Verification items for the finished model (mm, model axes). A direction names the side the tool comes from. Round coordinates to 2 decimals unless told otherwise and drop trailing zeros. Order: outer loops, then holes, each group sorted by start corner. A loop starts at its lowest first (then second) coordinate and runs counter-clockwise, first axis right, second up. Notation, with made-up numbers: (46.25, -11.5) -> (63.25, -11.5) arc R9 ccw to (63.25, 1.5) -> close; hole circle Ø3 at (20, 28). An arc over 180 degrees is marked (long way). Return JSON: item names as keys, results as strings. Group by question number.
Item 1: Access from +Z, -Z, +X, -X, +Y, -Y to the whole of each face (thin tool, end or side, straight path). Record for faces 1 (the cylindrical face through (-48, 18, 0)), 2 (the flat face through (20, 0, 0)), 3 (the flat face through (38, 13, 0)), 4 (the flat face through (-35.2, 13, 0.3)), 5 (the cylindrical face through (-22.5, 23, 0.1)).
Item 2: Sectioned sample at B-B on y = 21. Record the cut outline in (x, z), plus the area to 3 significant figures.
Item 3: Depth check by flat-ended pin: pin 1 Ø6.5 at (x, z) = (-31, 0) entering from -Y; pin 2 Ø4 at (y, z) = (6.5, 5.5) entering from -X; pin 3 Ø6.5 at (y, z) = (6, -3.5) entering from +X; pin 4 Ø5.5 at (x, z) = (0, 0) entering from +Y (3 decimals). Enter the tip coordinate at first touch or a pass-through.
Item 4: Sectioned sample at A-A on x = 31. Record the cut outline in (y, z), plus the area to 3 significant figures.
Item 5: Sectioned sample at C-C on y = 7.5. Record the cut outline in (x, z), plus the area to 3 significant figures.
Item 6: Draft check along X on faces 6 (the cylindrical face through (2.93, 25.59, -0.65)), 7 (the cylindrical face through (22.5, 23, 0.1)), 8 (the flat face through (-38, 22, 0)). Enter one of: pulls with the +X half, pulls with the -X half, needs draft (parallel to the pull), parting line crosses it, or undercut.
Item 7: Sectioned sample at D-D on z = 0. Give the number of separate pieces and of enclosed holes in the cut face, plus the area to 3 significant figures.
Item 8: Scan lines: probe 1 along Z at (x, y) = (-31, 16); probe 2 along X at (y, z) = (24.25, 0); probe 3 along Y at (x, z) = (40.5, 1). Record each from-to range of solid material in increasing order. Write a range as from..to.
```python
from build123d import *

# Parameters (mm, degrees)
BOSS_EXTRUDE1_DEPTH   = 18
F_8_0MM_DOWEL_HOLE1_D = 8
CUT_EXTRUDE1_DEPTH    = 36
CUT_EXTRUDE4_DEPTH    = 36


with BuildPart() as part:
    # Sketch2 → Boss-Extrude1 (new body, symmetric)
    with BuildSketch(Plane.XY):
        with BuildLine():
            Line((18.027756377, 0), (22, 0))
            Line((22, 0), (22, 13))
            Line((22, 13), (50, 13))
            Line((50, 13), (50, 22))
            Line((50, 22), (25.690465157, 22))
            ThreePointArc((25.690465157, 22), (0, 32), (-25.690465157, 22))
            Line((-25.690465157, 22), (-50, 22))
            Line((-50, 22), (-50, 13))
            Line((-50, 13), (-22, 13))
            Line((-22, 13), (-22, 0))
            Line((-22, 0), (-18.027756377, 0))
            ThreePointArc((-18.027756377, 0), (0, 13), (18.027756377, 0))
        make_face()
    extrude(amount=BOSS_EXTRUDE1_DEPTH, both=True)

    # Ø8.0mm Dowel Hole1 (through all)
    with Locations(Plane(origin=(0, 22, 0), x_dir=(1, 0, 0), z_dir=(0, 1, 0))):
        with Locations((-31, 0)):
            f_8_0mm_dowel_hole1 = Hole(F_8_0MM_DOWEL_HOLE1_D / 2)

    # Sketch9 → Cut-Extrude1 (cut)
    with BuildSketch(Plane(origin=(0, 22, 0), x_dir=(1, 0, 0), z_dir=(0, 1, 0))):
        with BuildLine():
            ThreePointArc((-44.497190923, -18), (-48, 0), (-44.497190923, 18))
            Line((-44.497190923, 18), (-50, 18))
            Line((-50, 18), (-50, -18))
            Line((-50, -18), (-44.497190923, -18))
        make_face()
    cut_extrude1 = extrude(amount=-CUT_EXTRUDE1_DEPTH, mode=Mode.SUBTRACT)

    # Mirror1: Ø8.0mm Dowel Hole1, Cut-Extrude1 across plane
    add(f_8_0mm_dowel_hole1.mirror(Plane(origin=(0, 0, 0), x_dir=(0, 0, 1), z_dir=(1, 0, 0))), mode=Mode.SUBTRACT)
    add(cut_extrude1.mirror(Plane(origin=(0, 0, 0), x_dir=(0, 0, 1), z_dir=(1, 0, 0))), mode=Mode.SUBTRACT)

    # Sketch10 → CBORE for M5 Hex Head Bolt1 (revolve, cut)
    with BuildSketch(Plane(origin=(0, 32, 0), x_dir=(0, 0, 1), z_dir=(1, 0, 0))):
        Polygon((0, 0), (0, 32), (2.5, 32), (2.5, 13.495), (2.995, 13), (3, 13), (3, 0), align=None)
    revolve(axis=Axis((0, 38.35, 0), (0, -1, 0)), mode=Mode.SUBTRACT)

    # Sketch12 → Cut-Extrude4 (cut)
    with BuildSketch(Plane(origin=(0, 22, 0), x_dir=(1, 0, 0), z_dir=(0, 1, 0))):
        with BuildLine():
            Line((-25.690465157, 6.637683312), (-25.690465157, -6.637683312))
            ThreePointArc((-25.690465157, -6.637683312), (-22.5, 0), (-25.690465157, 6.637683312))
        make_face()
    cut_extrude4 = extrude(amount=CUT_EXTRUDE4_DEPTH, mode=Mode.SUBTRACT)

    # Mirror2: Cut-Extrude4 across plane
    add(cut_extrude4.mirror(Plane(origin=(0, 0, 0), x_dir=(0, 0, 1), z_dir=(1, 0, 0))), mode=Mode.SUBTRACT)


solid = part.part
```
Recorded:
{
 "1": {"face 1": "-X, +Y, -Y", "face 2": "+Z, -Z, +X, -X, -Y", "face 3": "+Z, -Z, +X, -Y", "face 4": "+Z, -Z, -X, -Y", "face 5": "-X, +Y"},
 "2": {"outline": "(-44.5, -18) -> (44.5, -18) arc R48 ccw to (44.5, 18) -> (-44.5, 18) arc R48 ccw to start; hole circle Ø8 at (-31, 0); hole circle Ø6 at (0, 0); hole circle Ø8 at (31, 0)", "area": "3,240 mm²"},
 "3": {"pin 1": "through", "pin 2": "x = -22", "pin 3": "x = 22", "pin 4": "y = 18.755"},
 "4": {"outline": "(13, -18) -> (22, -18) -> (22, -4) -> (13, -4) -> close; (13, 4) -> (22, 4) -> (22, 18) -> (13, 18) -> close", "area": "252 mm²"},
 "5": {"outline": "(-22, -18) -> (-13.37, -18) -> (-13.37, 18) -> (-22, 18) -> close; (13.37, -18) -> (22, -18) -> (22, 18) -> (13.37, 18) -> close", "area": "621 mm²"},
 "6": {"face 6": "undercut", "face 7": "pulls with the +X half", "face 8": "needs draft"},
 "7": {"separate pieces": "4", "enclosed holes": "0", "area": "1,180 mm²"},
 "8": {"probe 1": "-18..-4, 4..18", "probe 2": "-22.5..-3, 3..22.5", "probe 3": "13..22"}
}
